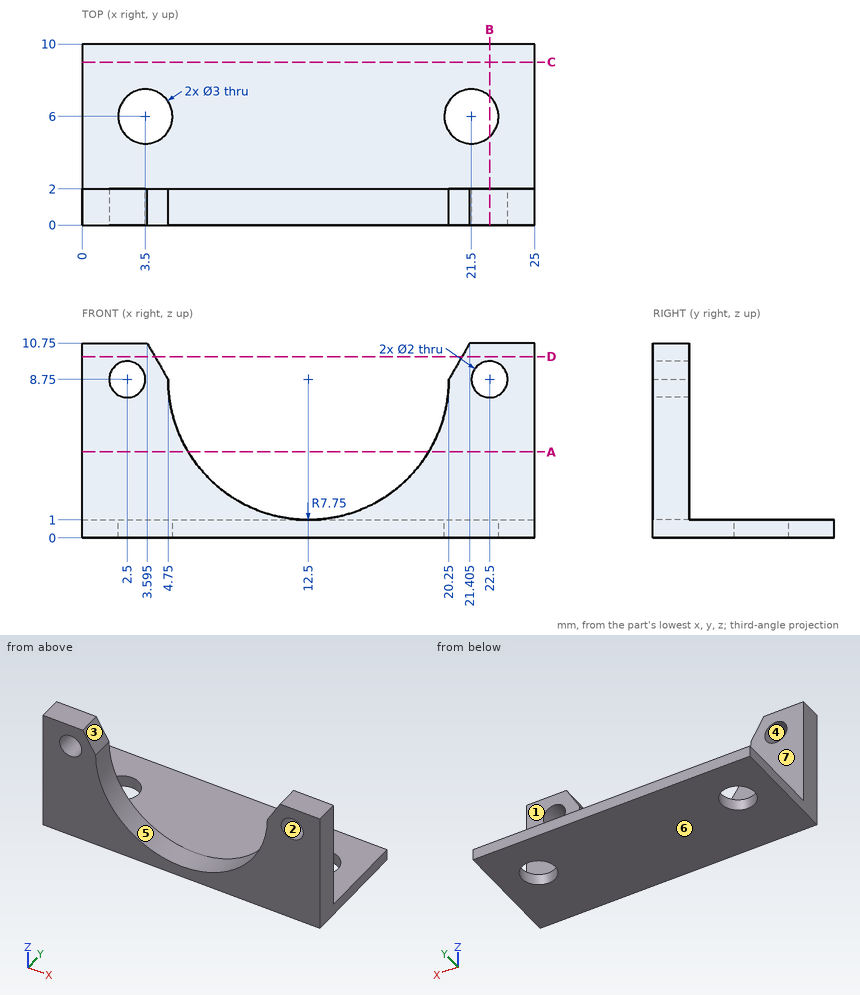
Geometry: see drawing. Coordinates: mm, zero at the bounding-box minimum. A direction names the side the tool comes from. Give positions to 0.01 mm unless a question says otherwise; leave off trailing zeros. Order: outer loops, then holes, each group sorted by start corner. A loop starts at its lowest first (then second) coordinate and runs counter-clockwise, first axis right, second up.
1. Cut plane D-D (z = 10). Return loops of the section in (x, y), and give its area (3 significant figures).
Computed:
outline: (0, 0) - (4.03, 0) - (4.03, 2) - (0, 2) - close; (20.97, 0) - (25, 0) - (25, 2) - (20.97, 2) - close
area: 16.1 mm2
2. Draft query along Z for the marked faces 4, 5, 6 and 7. Return one class per face: released by +Z, released by -Z, zero draft, split by the parting line, or undercut.
Computed:
face 4: undercut
face 5: released by +Z
face 6: released by -Z
face 7: zero draft
3. Line query: probe 1 along X at (y, z) = (6, 0.4); probe 2 along Z at (x, y) = (2.5, 1.45); probe 3 along Y at (x, z) = (21.5, 0.75). Output: solid intervals per line, ascending.
Computed:
probe 1: x = 0 to 2, 5 to 20, 23 to 25
probe 2: z = 0 to 7.75, 9.75 to 10.75
probe 3: y = 0 to 4.5, 7.5 to 10
4. Pin query (flat end, axial travel): pin 1 Ø4 at (y, z) = (5, 6) entering from +X; pin 2 Ø3.5 at (x, y) = (3.5, 6) entering from +Z; pin 3 Ø4 at (x, z) = (7.5, 2.5) entering from +Y; pin 4 Ø2.5 at (x, z) = (22.5, 8.75) entering from +Y. Return the tip coordinate at first contact, or that it passes through.
Computed:
pin 1: passes through
pin 2: stops at z = 1
pin 3: stops at y = 10
pin 4: stops at y = 2
5. Cut plane C-C (y = 9). Return loops of the section in (x, z), and give its area (3 significant figures).
Computed:
outline: (0, 0) - (25, 0) - (25, 1) - (0, 1) - close
area: 25.0 mm2
6. Cut plane B-B (x = 22.5). Return loops of the section in (y, z).
Computed:
outline: (0, 0) - (4.88, 0) - (4.88, 1) - (2, 1) - (2, 7.75) - (0, 7.75) - close; (0, 9.75) - (2, 9.75) - (2, 10.75) - (0, 10.75) - close; (7.12, 0) - (10, 0) - (10, 1) - (7.12, 1) - close
7. Set-up query: the marked faces 1, 2 and 3. Return all of +Z, -Z, +X, -X, +Y, -Y with unobstructed straight access to the full face (end or side cutting, diameter ignored); none if empty.
Computed:
face 1: +Z, +X, -X, +Y
face 2: +Y, -Y
face 3: +Z, +Y, -Y
8. Cut plane A-A (z = 4.75). Return loops of the section in (x, y).
Computed:
outline: (0, 0) - (5.86, 0) - (5.86, 2) - (0, 2) - close; (19.14, 0) - (25, 0) - (25, 2) - (19.14, 2) - close
